from build123d import *

# Parameters (mm, degrees)
EXTRUDE_1_DEPTH     = 1.24
CUT_EXTRUDE_1_DEPTH = 1.24
SKETCH_4_W          = 8.4
SKETCH_4_H          = 3
EXTRUDE_2_DEPTH     = 2.2
CHAMFER_1_SIZE      = 1.2
CHAMFER_1_SIZE_2    = 2.4
SKETCH_5_W          = 8.4
SKETCH_5_H          = 4.2
CUT_EXTRUDE_2_DEPTH = 23.25946091
SKETCH_6_W          = 8.4
SKETCH_6_H          = 3
EXTRUDE_3_DEPTH     = 2
CHAMFER_2_SIZE      = 2
CUT_EXTRUDE_3_DEPTH = 0.1


# Some blends are built 0.0001 mm under size
with BuildPart() as part:
    # Эскиз1 → Бобышка-Вытянуть1 (new body)
    with BuildSketch(Plane.XY):
        with BuildLine():
            Line((-4.6, 0), (-4.6, 6.174949393))
            ThreePointArc((-4.6, 6.174949393), (-6.88149693, 3.454706934), (-7.7, 0))
            Line((-7.7, 0), (-7.7, -20.6))
            Line((-7.7, -20.6), (7.7, -20.6))
            Line((7.7, -20.6), (7.7, 0))
            ThreePointArc((7.7, 0), (6.88149693, 3.454706934), (4.6, 6.174949393))
            Line((4.6, 6.174949393), (4.6, 0))
            ThreePointArc((4.6, 0), (0, -4.6), (-4.6, 0))
        make_face()
    extrude(amount=EXTRUDE_1_DEPTH)

    # Эскиз3 → Вырез-Вытянуть1 (cut)
    with BuildSketch(Plane.XY.offset(1.24)):
        with BuildLine():
            Line((-7.7, -20.6), (-4.2, -20.6))
            Line((-4.2, -20.6), (-4.2, -15.2))
            ThreePointArc((-4.2, -15.2), (-5.1372583, -12.9372583), (-7.4, -12))
            Line((-7.4, -12), (-7.7, -12))
            Line((-7.7, -12), (-7.7, -20.6))
        make_face()
        with BuildLine():
            Line((4.2, -20.6), (4.2, -15.2))
            ThreePointArc((4.2, -15.2), (5.1372583, -12.9372583), (7.4, -12))
            Line((7.4, -12), (7.7, -12))
            Line((7.7, -12), (7.7, -20.6))
            Line((7.7, -20.6), (4.2, -20.6))
        make_face()
    extrude(amount=-CUT_EXTRUDE_1_DEPTH, mode=Mode.SUBTRACT)

    # Эскиз4 → Бобышка-Вытянуть2 (add)
    with BuildSketch(Plane.XY.offset(1.24)):
        with Locations((0, -19.1)):
            Rectangle(SKETCH_4_W, SKETCH_4_H)
    extrude(amount=EXTRUDE_2_DEPTH)

    # Фаска1
    # the kernel refuses this chamfer: 2.4, 1.2 mm, written as the material it adds along each edge
    with BuildSketch(Plane(origin=(4.2, -17.6, 1.24), x_dir=(0, 0.9976223042390325, -0.06891834360170876), z_dir=(-1, 0, 0))) as chamfer_1_piece_1_section:
        Polygon((CHAMFER_1_SIZE * 0.997622304239, -CHAMFER_1_SIZE * 0.0689183436017), (-CHAMFER_1_SIZE_2 * 0.0689183436017, -CHAMFER_1_SIZE_2 * 0.997622304239), (0, 0), align=None)
    chamfer_1_piece_1 = extrude(amount=8.4, mode=Mode.PRIVATE)
    chamfer_1_piece_1 = split(chamfer_1_piece_1, bisect_by=Plane(origin=(0, -17.211387721, 3.44), z_dir=(0, 0, -1)), keep=Keep.TOP, mode=Mode.PRIVATE)
    add(chamfer_1_piece_1)

    # Эскиз5 → Вырез-Вытянуть2 (cut, through all)
    with BuildSketch(Plane.XY.offset(3.44)):
        with Locations((0, -18.5)):
            Rectangle(SKETCH_5_W, SKETCH_5_H)
    extrude(amount=-CUT_EXTRUDE_2_DEPTH, mode=Mode.SUBTRACT)

    # Эскиз6 → Бобышка-Вытянуть3 (add)
    with BuildSketch(Plane.XY.offset(1.24)):
        with Locations((0, -14.9)):
            Rectangle(SKETCH_6_W, SKETCH_6_H)
    extrude(amount=EXTRUDE_3_DEPTH)

    # Фаска2
    chamfer_2_edges = [part.edges().sort_by_distance(p)[0] for p in [
        (0, -13.4, 3.24),
    ]]
    chamfer(chamfer_2_edges, length=CHAMFER_2_SIZE - 0.0001)  # a hair under: the kernel refuses the full size

    # Эскиз7 → Вырез-Вытянуть3 (cut)
    with BuildSketch(Plane(origin=(0, 0, 0), x_dir=(-1, 0, 0), z_dir=(0, 0, -1))):
        with BuildLine():
            Line((-4.2, -15.2), (-4.2, -16.4))
            Line((-4.2, -16.4), (4.2, -16.4))
            Line((4.2, -16.4), (4.2, -15.2))
            ThreePointArc((4.2, -15.2), (5.1372583, -12.9372583), (7.4, -12))
            Line((7.4, -12), (7.7, -12))
            Line((7.7, -12), (7.7, 0))
            ThreePointArc((7.7, 0), (6.88149693, 3.454706934), (4.6, 6.174949393))
            Line((4.6, 6.174949393), (4.6, 0))
            ThreePointArc((4.6, 0), (0, -4.6), (-4.6, 0))
            Line((-4.6, 0), (-4.6, 6.174949393))
            ThreePointArc((-4.6, 6.174949393), (-6.88149693, 3.454706934), (-7.7, 0))
            Line((-7.7, 0), (-7.7, -12))
            Line((-7.7, -12), (-7.4, -12))
            ThreePointArc((-7.4, -12), (-5.1372583, -12.9372583), (-4.2, -15.2))
        make_face()
    extrude(amount=-CUT_EXTRUDE_3_DEPTH, mode=Mode.SUBTRACT)


solid = part.part
For this review, take the finished solid that the model builds, in its own axes (mm). A direction names the side the tool comes from. Give positions to 0.01 mm unless a question says otherwise; leave off trailing zeros. Loops run counter-clockwise (first coordinate to the right, second up) from the corner with the lowest first, then second, coordinate; pieces in that order, holes last. Notation, with made-up numbers: M 59.25,-9.75 L 68.25,-9.75 A23 ccw 68.25,1.25 Z; hole C 32,-0.75 d5. An arc over 180 degrees is marked long. Put each result on its own line as item: value. Start each with the question number.
(1) Wall thickness on L1, parallel to X at y = -3.25, z = 0.5; L2, parallel to Z at x = 3.5, y = -7; L3, parallel to X at y = 0.5, z = 0.8: over which ranges is each line inside the solid? List them lowest first.
(2) The part is to be moulded in two halves that separate along X. For faces 6 (the flat face through (0, -7, 1.24)), 7 (the cylindrical face through (-5.113, -12.962, 0.678)), 8 (the cylindrical face through (0.1, -4.6, 0.7)), 9 (the flat face through (7.7, -6, 1)), say which applies: +X half, -X half, draft (parallel to the pull), parting line (faces both ways), or undercut.
(3) Machinability: for faces 1 (the flat face through (4.6, 3, 1)), 2 (the flat face through (-4.2, -15, 2)), 3 (the flat face through (4.2, -15, 2)), 4 (the cylindrical face through (-6.86, 3.5, 0.66)), 5 (the flat face through (0, -16, 3.24)), which of the approach directions +Z, -Z, +X, -X, +Y, -Y give a long, thin tool a straight path to every point of the face, cutting with its end or side? Answer none if there is none.
(4) Add section A-A, the plane z = 0.6. Write out the cut boundary in (x, y).
(5) For pin 1 (0.9 mm diameter, centred on y = 2, z = 1, fed in from +X); pin 2 (8 mm diameter, centred on x = 2.5, y = 2.5, fed in from +Z); pin 3 (8 mm diameter, centred on x = -3.5, y = -11, fed in from +Z), all flat-tipped, find the tip position at first contact; note any pin that passes through.
(6) Add section B-B, the plane y = 2.5. Write out the cut boundary in (x, z), then the cut area to 3 significant figures.
Result:
1. L1: x = -7.7 to -3.26, 3.26 to 7.7
1. L2: z = 0.1 to 1.24
1. L3: x = -7.68 to -4.6, 4.6 to 7.68
2. face 6: draft
2. face 7: -X half
2. face 8: undercut
2. face 9: +X half
3. face 1: +Z, -Z, +Y
3. face 2: +Z, -X, -Y
3. face 3: +Z, +X, -Y
3. face 4: +Z, -Z, -X, +Y
3. face 5: +Z, +X, -X, +Y, -Y
4. outline: M -7.7,-12 L -7.4,-12 A3.2 cw -4.2,-15.2 L -4.2,-16.4 L 4.2,-16.4 L 4.2,-15.2 A3.2 cw 7.4,-12 L 7.7,-12 L 7.7,0 A7.7 ccw 4.6,6.17 L 4.6,0 A4.6 cw -4.6,0 L -4.6,6.17 A7.7 ccw -7.7,0 Z
5. pin 1: stops at x = 7.54
5. pin 2: stops at z = 1.24
5. pin 3: stops at z = 2.84
6. outline: M -7.28,0.1 L -4.6,0.1 L -4.6,1.24 L -7.28,1.24 Z; M 4.6,0.1 L 7.28,0.1 L 7.28,1.24 L 4.6,1.24 Z
6. area: 6.12 mm^2
